Read the model definition and answer for the solid it produces. Units are mm, in the model's axes. Give positions to 0.01 mm unless a question says otherwise; leave off trailing zeros. Order: outer loops, then holes, each group sorted by start corner. A loop starts at its lowest first (then second) coordinate and runs counter-clockwise, first axis right, second up. Notation, with made-up numbers: (-28.5, 73) - (22.5, 73) arc R8 ccw to (22.5, 77) - close; hole circle Ø4 at (14, -24.75). An arc over 180 degrees is marked (long way). Answer as CSV lines item,"result". Start each with the question number.
from build123d import *

# Parameters (mm, degrees)
SKETCH_1_R          = 1.6
EXTRUDE_1_DEPTH     = 2
CUT_EXTRUDE_1_DEPTH = 161.623784042
CHAMFER_1_SIZE      = 0.2
CHAMFER_1_SIZE2     = 0.1
CHAMFER_2_SIZE2     = 0.2
CHAMFER_2_SIZE      = 0.1


with BuildPart() as part:
    # Эскиз1 → Бобышка-Вытянуть1 (new body)
    # profile 1 of 3: a face of its own
    with BuildSketch(Plane(origin=(0, 0, 0), x_dir=(1, 0, 0), z_dir=(0, 1, 0))):
        with BuildLine():
            Line((75, 14), (-75, 14))
            Line((-75, 14), (-75, 1.6))
            ThreePointArc((-75, 1.6), (-73.86862915, 1.13137085), (-73.4, 0))
            ThreePointArc((-73.4, 0), (-73.86862915, -1.13137085), (-75, -1.6))
            Line((-75, -1.6), (-75, -14))
            Line((-75, -14), (75, -14))
            Line((75, -14), (75, -1.6))
            ThreePointArc((75, -1.6), (73.4, 0), (75, 1.6))
            Line((75, 1.6), (75, 14))
        make_face()
        with Locations(Location((-25, 0, 0), (0, 0, 270))):
            Circle(SKETCH_1_R, mode=Mode.SUBTRACT)
        with Locations(Location((25, 0, 0), (0, 0, 270))):
            Circle(SKETCH_1_R, mode=Mode.SUBTRACT)
    # profile 2 of 3: a face of its own
    with BuildSketch(Plane(origin=(0, 0, 0), x_dir=(1, 0, 0), z_dir=(0, 1, 0))):
        with BuildLine():
            Line((79.670248868, 1.785714286), (75, 14))
            Line((75, 14), (75, 1.6))
            ThreePointArc((75, 1.6), (76.13137085, 1.13137085), (76.6, 0))
            ThreePointArc((76.6, 0), (76.13137085, -1.13137085), (75, -1.6))
            Line((75, -1.6), (75, -14))
            Line((75, -14), (79.670248868, -1.785714286))
            ThreePointArc((79.670248868, -1.785714286), (80, 0), (79.670248868, 1.785714286))
        make_face()
    # profile 3 of 3: a face of its own
    with BuildSketch(Plane(origin=(0, 0, 0), x_dir=(1, 0, 0), z_dir=(0, 1, 0))):
        with BuildLine():
            Line((-75, 1.6), (-75, 14))
            Line((-75, 14), (-79.670248868, 1.785714286))
            ThreePointArc((-79.670248868, 1.785714286), (-80, 0), (-79.670248868, -1.785714286))
            Line((-79.670248868, -1.785714286), (-75, -14))
            Line((-75, -14), (-75, -1.6))
            ThreePointArc((-75, -1.6), (-76.6, 0), (-75, 1.6))
        make_face()
    extrude(amount=EXTRUDE_1_DEPTH)

    # Эскиз3 → Вырез-Вытянуть1 (cut, through all)
    with BuildSketch(Plane.ZY.offset(80)):
        Polygon((-12.645299462, 0), (-14, 0), (-14, 2), (-13.8, 2), align=None)
        Polygon((14, 0), (14, 2), (13.8, 2), (12.645299462, 0), align=None)
    extrude(amount=-CUT_EXTRUDE_1_DEPTH, mode=Mode.SUBTRACT)

    # Фаска1
    chamfer_1_edges = [part.edges().sort_by_distance(p)[0] for p in [
        (0, 2, -13.8),
    ]]
    chamfer_1_side = [part.faces().sort_by_distance(p)[0] for p in [
        (0, 0.999022738, -13.222085508),
    ]]
    chamfer(chamfer_1_edges, length=CHAMFER_1_SIZE, length2=CHAMFER_1_SIZE2, reference=chamfer_1_side[0])

    # Фаска2
    chamfer_2_edges = [part.edges().sort_by_distance(p)[0] for p in [
        (0, 2, 13.8),
    ]]
    chamfer_2_side = [part.faces().sort_by_distance(p)[0] for p in [
        (0, 2, 13.798),
    ]]
    chamfer(chamfer_2_edges, length=CHAMFER_2_SIZE - 0.0001, length2=CHAMFER_2_SIZE2 - 0.0001, reference=chamfer_2_side[0])  # a hair under: the kernel refuses the full size


solid = part.part
(1) Straight lines are drawn through the part: line 1 (X direction, y = 1.65, z = 1.75); line 2 (X direction, y = 1.45, z = -1.25); line 3 (X direction, y = 1.25, z = 4.75). For each, find the intervals that lie inside material, in ascending order. Write a range as [from, to].
(2) Flat-ended cylindrical pins translate along their axes: pin 1 Ø4 at (x, z) = (-16, -10.5) entering from -Y; pin 2 Ø1 at (y, z) = (0.5, 8.5) entering from +X. Find the tip coordinate at first contact, or state that the pin passes through.
(3) Section C-C, the plane x = 60.5 is taken. Write down the section's boundary in (y, z), and give its area (3 significant figures).
(4) Section B-B, the plane y = 1.1 is taken. Write down the section's boundary in (x, z), and give its area (3 significant figures).
(5) Section A-A, the plane x = 25 is taken. Write down the section's boundary in (y, z).
(6) Section D-D, the plane z = 9.75 is taken. Write down the section's boundary in (x, y).
(7) Determine the mould class of faces 1 (the flat face through (-1, 2, 0)), 2 (the flat face through (-77.36, 0.99, -7.83)), 3 (the flat face through (77.36, 0.99, 7.83)), 4 (the cylindrical face through (24.03, 0.99, -1.27)) for opening direction X: released by +X, released by -X, zero draft, split by the parting line, or undercut.
Checks:
1,line 1,"x = [-79.68, 79.68]"
1,line 2,"x = [-79.84, -76], [-74, -26], [-24, 24], [26, 74], [76, 79.84]"
1,line 3,"x = [-78.54, 78.54]"
2,pin 1,"stops at y = 0"
2,pin 2,"stops at x = 77.29"
3,outline,"(0, -12.65) - (1.83, -13.7) - (2, -13.7) - (2, 13.7) - (1.83, 13.7) - (0, 12.65) - close"
3,area,"52.9 mm²"
4,outline,"(-79.67, -1.79) - (-75.28, -13.28) - (75.28, -13.28) - (79.67, -1.79) arc R5 ccw to (79.67, 1.79) - (75.28, 13.28) - (-75.28, 13.28) - (-79.67, 1.79) arc R5 ccw to start; hole circle Ø3.2 at (-75, 0); hole circle Ø3.2 at (-25, 0); hole circle Ø3.2 at (25, 0); hole circle Ø3.2 at (75, 0)"
4,area,"4,100 mm²"
5,outline,"(0, -12.65) - (1.83, -13.7) - (2, -13.7) - (2, -1.6) - (0, -1.6) - close; (0, 1.6) - (2, 1.6) - (2, 13.7) - (1.83, 13.7) - (0, 12.65) - close"
6,outline,"(-76.63, 0) - (76.63, 0) - (76.63, 2) - (-76.63, 2) - close"
7,face 1,"zero draft"
7,face 2,"released by -X"
7,face 3,"released by +X"
7,face 4,"undercut"
